The listing builds one solid part. Answer for the finished solid, in the listing's coordinates (mm). A direction names the side the tool comes from. Give positions to 0.01 mm unless a question says otherwise; leave off trailing zeros. Loops run counter-clockwise (first coordinate to the right, second up) from the corner with the lowest first, then second, coordinate; pieces in that order, holes last. Notation, with made-up numbers: (25, -4.75) - (53, -4.75) arc R11 ccw to (53, 15.25) - close; hole circle Ø7 at (70.25, 42.5). An arc over 180 degrees is marked (long way). Write item = value, one per line. Start each with the question number.
1) The part is cut by section C-C on y = -2. Write down the section's boundary in (x, z).
2) The part is cut by section A-A on x = -14.6. Write down the section's boundary in (y, z), plus the area to 3 significant figures.
3) The part is cut by section D-D on x = 1. Write down the section's boundary in (y, z), plus the area to 3 significant figures.
4) Flat-ended cylindrical pins translate along their axes: P1, Ø0.5, axis at x = -21.5, y = 2.5, coming from the -Z side; P2, Ø0.8, axis at y = 2.5, z = 16, coming from the +X side; P3, Ø10, axis at x = -11, z = 33.5, coming from the -Y side. Find the tip coordinate at first contact, or state that the pin passes through.
5) Which of the six approach directions +Z, -Z, +X, -X, +Y, -Y give full straight-line access (tool end or side, diameter ignored) to faces 1 (the flat face through (5, -4, 14)), 2 (the flat face through (-8, -1, 16))?
6) The mould has two halves that part along X. Classify faces 3 (the cylindrical face through (-14.66, 2.48, 14.8)), 4 (the flat face through (25.4, -2, 25)), 5 (the flat face through (-25.4, 2.2, 18.1)), 6 (the flat face through (0, -1, 0)): +X half, -X half, draft (parallel to the pull), parting line (faces both ways), or undercut.
7) The part is cut by section B-B on z = 23.18. Write down the section's boundary in (x, y).
8) Consider probe 1 along Z at (x, y) = (12.7, -1.6); probe 2 along X at (y, z) = (-0.4, 43.18); probe 3 along X at (y, z) = (-0.15, 12.7). Determine where each line is inside the solid, lowest interval first.
from build123d import *

# Parameters (mm, degrees)
SKETCH1_W           = 50.8
SKETCH1_H           = 8
BOSS_EXTRUDE1_DEPTH = 50.8
SKETCH2_W           = 34.8
SKETCH2_H           = 5
CUT_EXTRUDE2_DEPTH  = 34.8
CUT_EXTRUDE3_DEPTH  = 3
FILLET1_R           = 1
SKETCH4_R           = 2.1
CUT_EXTRUDE4_DEPTH  = 4
SKETCH5_R           = 1.65
CUT_EXTRUDE5_DEPTH  = 6


with BuildPart() as part:
    # Sketch1 → Boss-Extrude1 (new body)
    with BuildSketch(Plane.XY):
        Rectangle(SKETCH1_W, SKETCH1_H)
    extrude(amount=BOSS_EXTRUDE1_DEPTH)

    # Sketch2 → Cut-Extrude2 (cut)
    with BuildSketch(Plane.XY.offset(50.8)):
        with Locations((-8, -1.5)):
            Rectangle(SKETCH2_W, SKETCH2_H)
    extrude(amount=-CUT_EXTRUDE2_DEPTH, mode=Mode.SUBTRACT)

    # Sketch3 → Cut-Extrude3 (cut)
    with BuildSketch(Plane(origin=(0, 4, 0), x_dir=(1, 0, 0), z_dir=(0, 1, 0))):
        Polygon((-25.4, -12.7), (12.7, -12.7), (12.7, -50.8), (25.4, -50.8), (25.4, 0), (-25.4, 0), align=None)
    extrude(amount=-CUT_EXTRUDE3_DEPTH, mode=Mode.SUBTRACT)

    # Fillet1
    fillet1_edges = [part.edges().sort_by_distance(p)[0] for p in [
        (-25.4, 2.5, 50.8),
        (17.4, -4, 50.8),
        (-25.4, -4, 8),
        (9.4, -1.5, 50.8),
        (-8, 1, 50.8),
        (-8, -4, 16),
        (9.4, -4, 33.4),
        (9.4, -1.5, 16),
        (9.4, 1, 33.4),
        (-8, 1, 16),
        (-25.4, 1, 33.4),
        (-25.4, -1.5, 16),
        (-25.4, -1.5, 0),
        (-6.35, 4, 50.8),
        (-25.4, 2.5, 12.7),
        (12.7, 2.5, 50.8),
        (-6.35, 4, 12.7),
        (12.7, 4, 31.75),
        (-25.4, 1, 6.35),
        (0, 1, 0),
        (25.4, 1, 25.4),
        (19.05, 1, 50.8),
        (12.7, 1, 31.75),
        (-6.35, 1, 12.7),
        (25.4, -1.5, 50.8),
        (0, -4, 0),
        (25.4, -1.5, 0),
        (25.4, -4, 25.4),
        (-25.4, 4, 31.75),
    ]]
    fillet(fillet1_edges, radius=FILLET1_R)

    # Sketch4 → Cut-Extrude4 (cut, through all)
    with BuildSketch(Plane(origin=(0, 1, 0), x_dir=(1, 0, 0), z_dir=(0, 1, 0))):
        with Locations((-14.6, -12.7)):
            Circle(SKETCH4_R)
        with Locations((12.7, -43.18)):
            Circle(SKETCH4_R)
        with Locations((12.7, -23.18)):
            Circle(SKETCH4_R)
    extrude(amount=CUT_EXTRUDE4_DEPTH, mode=Mode.SUBTRACT)

    # Sketch5 → Cut-Extrude5 (cut, through all)
    with BuildSketch(Plane(origin=(0, 1, 0), x_dir=(1, 0, 0), z_dir=(0, 1, 0))):
        with Locations((-14.6, -12.7)):
            Circle(SKETCH5_R)
        with Locations((12.7, -23.18)):
            Circle(SKETCH5_R)
        with Locations((12.7, -43.18)):
            Circle(SKETCH5_R)
    extrude(amount=-CUT_EXTRUDE5_DEPTH, mode=Mode.SUBTRACT)


solid = part.part
Answer below:
q1.outline = (-25.4, 1) arc R1 ccw to (-24.4, 0) - (24.4, 0) arc R1 ccw to (25.4, 1) - (25.4, 49.8) arc R1 ccw to (24.4, 50.8) - (10.4, 50.8) arc R1 ccw to (9.4, 49.8) - (9.4, 17) arc R1 cw to (8.4, 16) - (-24.4, 16) arc R1 ccw to (-25.4, 15) - close; hole circle Ø3.3 at (-14.6, 12.7); hole circle Ø3.3 at (12.7, 23.18); hole circle Ø3.3 at (12.7, 43.18)
q2.outline = (-4, 1) arc R1 ccw to (-3, 0) - (0, 0) arc R1 ccw to (1, 1) - (1, 11.05) - (-4, 11.05) - close; (-4, 14.35) - (1, 14.35) - (1, 14.8) - (4, 14.8) - (4, 49.8) arc R1 ccw to (3, 50.8) - (2, 50.8) arc R1 ccw to (1, 49.8) - (1, 17) arc R1 cw to (0, 16) - (-3, 16) arc R1 ccw to (-4, 15) - close
q2.area = 171 mm2
q3.outline = (-4, 1) arc R1 ccw to (-3, 0) - (0, 0) arc R1 ccw to (1, 1) - (1, 11.7) arc R1 cw to (2, 12.7) - (3, 12.7) arc R1 ccw to (4, 13.7) - (4, 49.8) arc R1 ccw to (3, 50.8) - (2, 50.8) arc R1 ccw to (1, 49.8) - (1, 17) arc R1 cw to (0, 16) - (-3, 16) arc R1 ccw to (-4, 15) - close
q3.area = 193 mm2
q4.P1 = 12.7
q4.P2 = 12.7
q4.P3 = 1
q5.face_1 = +Z, -Z, +X, -X, -Y
q5.face_2 = +Z, -X, -Y
q6.face_3 = undercut
q6.face_4 = +X half
q6.face_5 = -X half
q6.face_6 = draft
q7.outline = (-25.4, 2) arc R1 ccw to (-24.4, 1) - (8.4, 1) arc R1 cw to (9.4, 0) - (9.4, -3) arc R1 ccw to (10.4, -4) - (11.05, -4) - (11.05, 1) - (10.6, 1) - (10.6, 4) - (-24.4, 4) arc R1 ccw to (-25.4, 3) - close; (14.35, -4) - (24.4, -4) arc R1 ccw to (25.4, -3) - (25.4, 0) arc R1 ccw to (24.4, 1) - (14.35, 1) - close
q8.probe_1 = 0 to 21.53, 24.83 to 41.53, 44.83 to 50.8
q8.probe_2 = 9.4 to 11.05, 14.35 to 25.4
q8.probe_3 = -25.4 to -16.25, -12.95 to 25.4
